Could you check a few things on this model? Use its own coordinates, in mm. A direction names the side the tool comes from. Give positions to 0.01 mm unless a question says otherwise; leave off trailing zeros. Loops run counter-clockwise (first coordinate to the right, second up) from the corner with the lowest first, then second, coordinate; pieces in that order, holes last. Notation, with made-up numbers: (-6, 39) - (7, 39) arc R27 ccw to (7, 78) - close; hole circle Ø7 at (29.5, 56). An arc over 180 degrees is marked (long way). Write each question's results on one line, items separated by ' | '. Start each with the question number.
```python
from build123d import *

# Parameters (mm, degrees)
ESQUISSE1_W             = 46
ESQUISSE1_H             = 370
ESQUISSE1_W_2           = 8
ESQUISSE1_H_2           = 6
BOSS_EXTRU_1_DEPTH      = 6
ESQUISSE2_R             = 12.5
ESQUISSE2_R_2           = 5
ENL_V_MAT_EXTRU_1_DEPTH = 6
CONG_1_R                = 10


with BuildPart() as part:
    # Esquisse1 → Boss.-Extru.1 (new body)
    with BuildSketch(Plane.XY):
        with Locations((23, 185)):
            Rectangle(ESQUISSE1_W, ESQUISSE1_H)
        with Locations((23, 8)):
            Rectangle(ESQUISSE1_W_2, ESQUISSE1_H_2, mode=Mode.SUBTRACT)
        with Locations((23, 362)):
            Rectangle(ESQUISSE1_W_2, ESQUISSE1_H_2, mode=Mode.SUBTRACT)
    extrude(amount=BOSS_EXTRU_1_DEPTH)

    # Esquisse2 → Enlèv. mat.-Extru.1 (cut)
    with BuildSketch(Plane.XY.offset(6)):
        with Locations((30, 32)):
            Circle(ESQUISSE2_R)
        with Locations((30, 66)):
            Circle(ESQUISSE2_R)
        with Locations((30, 100)):
            Circle(ESQUISSE2_R)
        with Locations((30, 134)):
            Circle(ESQUISSE2_R)
        with Locations((30, 168)):
            Circle(ESQUISSE2_R)
        with Locations((30, 202)):
            Circle(ESQUISSE2_R)
        with Locations((30, 236)):
            Circle(ESQUISSE2_R)
        with Locations((30, 270)):
            Circle(ESQUISSE2_R)
        with Locations((30, 304)):
            Circle(ESQUISSE2_R)
        with Locations((8.281143203, 338)):
            Circle(ESQUISSE2_R_2)
        with Locations((8.281143203, 304)):
            Circle(ESQUISSE2_R_2)
        with Locations((8.281143203, 270)):
            Circle(ESQUISSE2_R_2)
        with Locations((8.281143203, 236)):
            Circle(ESQUISSE2_R_2)
        with Locations((8.281143203, 202)):
            Circle(ESQUISSE2_R_2)
        with Locations((8.281143203, 168)):
            Circle(ESQUISSE2_R_2)
        with Locations((8.281143203, 134)):
            Circle(ESQUISSE2_R_2)
        with Locations((8.281143203, 100)):
            Circle(ESQUISSE2_R_2)
        with Locations((8.281143203, 66)):
            Circle(ESQUISSE2_R_2)
        with Locations((30, 338)):
            Circle(ESQUISSE2_R)
        with Locations((8.281143203, 32)):
            Circle(ESQUISSE2_R_2)
    extrude(amount=-ENL_V_MAT_EXTRU_1_DEPTH, mode=Mode.SUBTRACT)

    # Congé1
    cong_1_edges = [part.edges().sort_by_distance(p)[0] for p in [
        (46, 370, 3),
        (46, 0, 3),
    ]]
    fillet(cong_1_edges, radius=CONG_1_R)


solid = part.part
```
Q1. I want a section at C-C, the plane y = 109.5. List the corners of the cut face in (x, z) for me.
Q2. I want a section at B-B, the plane y = 32. List the corners of the cut face in (x, z) for me, then the cut area to 3 significant figures.
Q3. Which directions (+Z, -Z, +X, -X, +Y, -Y) give clear straight access to the entire face, cutting with the end or side of a thin tool? Please do faces 4 (the face through (23, 188, 6)), 5 (the face through (27, 8, 3)).
Q4. I'm going to push a flat-ended pin straight in: pin 1 Ø2 at (y, z) = (49.5, 3.5) entering from -X. Where does the tip first touch, or does it pass through?
Q5. I want a section at A-A, the plane z = 1.45. State how many separate pieces and enclosed holes the cut face has, then the cut area to 3 significant figures.
Q6. I need wall thicknesses on L1, parallel to X at y = 237.5, z = 4.75; L2, parallel to X at y = 99, z = 0.35. Which ranges of each line are inside material? Lowest first, please. Write a range as from..to.
Q7. If we mould it in two halves opening along Y, with no side actions, what happens to faces 1 (the face through (42.99, 2.85, 3.04)), 2 (the face through (13.05, 101.5, 3.04)), 3 (the face through (42.99, 367.15, 3.04))? For each: +Y half, -Y half, draft (parallel to the pull), parting line (faces both ways), or undercut.
Conclusion:
1) outline: (0, 0) - (21.88, 0) - (21.88, 6) - (0, 6) - close; (38.12, 0) - (46, 0) - (46, 6) - (38.12, 6) - close
2) outline: (0, 0) - (3.28, 0) - (3.28, 6) - (0, 6) - close; (13.28, 0) - (17.5, 0) - (17.5, 6) - (13.28, 6) - close; (42.5, 0) - (46, 0) - (46, 6) - (42.5, 6) - close | area: 66.0 mm^2
3) face 4: +Z, +X, -X, +Y, -Y | face 5: +Z, -Z
4) pin 1: x = 0
5) separate pieces: 1 | enclosed holes: 22 | area: 11,200 mm^2
6) L1: 0..3.51, 13.05..17.59, 42.41..46 | L2: 0..3.38, 13.18..17.54, 42.46..46
7) face 1: -Y half | face 2: undercut | face 3: +Y half
